Could you check a few things on this drawing? It's one solid part, dimensions in mm from its lowest x, y, z. A direction names the side the tool comes from. Coordinates: 2 decimals unless noted, no trailing zeros. Write each loop counter-clockwise with the first axis right and the second up, starting at its lowest first coordinate (ties: lowest second). Pieces come first, ordered by that corner, then holes. Notation, with made-up numbers: M -1,32.25 L 4,32.25 A27 ccw 4,67.25 Z; hole C -16,-40 d2. An arc over 180 degrees is marked long. Use a Markdown table: item, result.
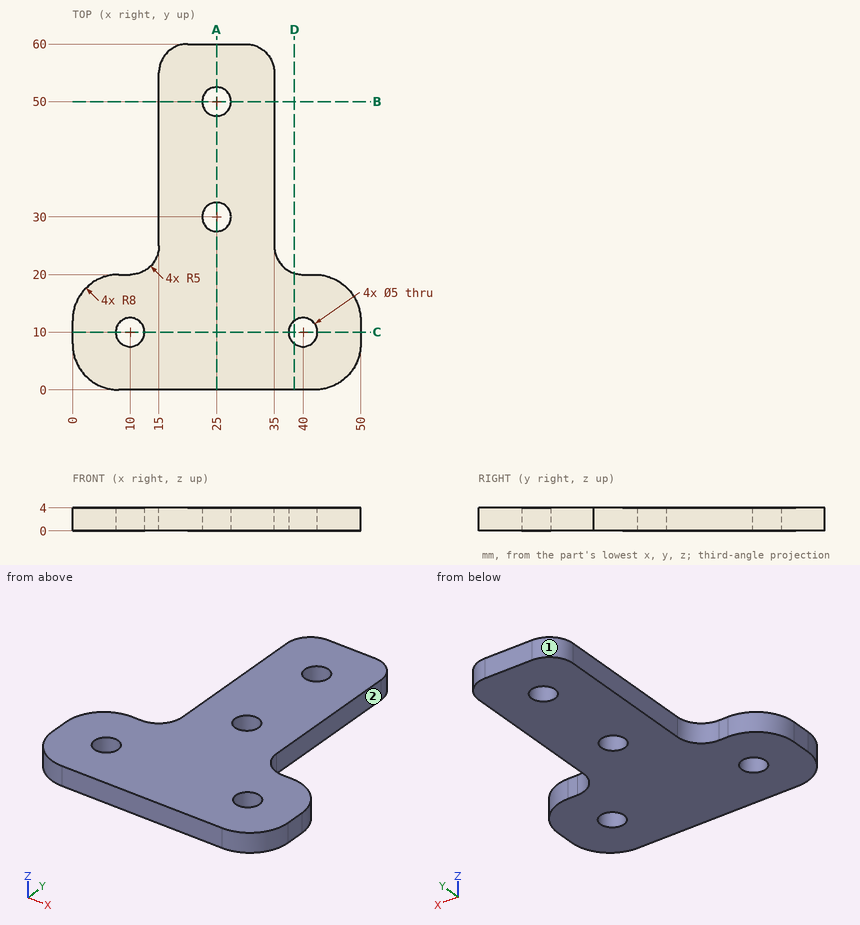
1. Suppose I cut it at B-B on y = 50. Write out the boundary of the cut face in (x, z), and give its area (3 significant figures).
Answers follow:
| item | result |
|---|---|
| outline | M 15,0 L 22.5,0 L 22.5,4 L 15,4 Z; M 27.5,0 L 35,0 L 35,4 L 27.5,4 Z |
| area | 60.0 mm2 |
2. Suppose I cut it at D-D on x = 38.5. Write out the boundary of the cut face in (y, z), and give its area (3 significant figures).
Answers follow:
| item | result |
|---|---|
| outline | M 0,0 L 8,0 L 8,4 L 0,4 Z; M 12,0 L 20.23,0 L 20.23,4 L 12,4 Z |
| area | 64.9 mm2 |
3. Which directions (+Z, -Z, +X, -X, +Y, -Y) give clear straight access to the entire face, cutting with the end or side of a thin tool? Please do the marked faces 1 and 2.
Answers follow:
| item | result |
|---|---|
| face 1 | +Z, -Z, -X, +Y |
| face 2 | +Z, -Z, +X, +Y |
4. Suppose I cut it at A-A on x = 25. Write out the boundary of the cut face in (y, z), and give its area (3 significant figures).
Answers follow:
| item | result |
|---|---|
| outline | M 0,0 L 27.5,0 L 27.5,4 L 0,4 Z; M 32.5,0 L 47.5,0 L 47.5,4 L 32.5,4 Z; M 52.5,0 L 60,0 L 60,4 L 52.5,4 Z |
| area | 200 mm2 |
5. I need wall thicknesses on probe 1 along Y at (x, z) = (25, 1.7); probe 2 along X at (y, z) = (25, 1.2); probe 3 along Y at (x, z) = (38, 1.65). Which ranges of each line are inside material? Lowest first, please.
Answers follow:
| item | result |
|---|---|
| probe 1 | y = 0 to 27.5, 32.5 to 47.5, 52.5 to 60 |
| probe 2 | x = 15 to 35 |
| probe 3 | y = 0 to 8.5, 11.5 to 20.42 |
6. Will these pins go through, and if not, where does the flat tip stop? pin 1 Ø4.5 at (x, y) = (10, 10) entering from -Z; pin 2 Ø0.6 at (x, z) = (8.5, 1) entering from +Y; pin 3 Ø2 at (y, z) = (39.5, 1.5) entering from +X.
Answers follow:
| item | result |
|---|---|
| pin 1 | passes through |
| pin 2 | stops at y = 20 |
| pin 3 | stops at x = 35 |
7. Suppose I cut it at C-C on y = 10. Write out the boundary of the cut face in (x, z), and give its area (3 significant figures).
Answers follow:
| item | result |
|---|---|
| outline | M 0,0 L 7.5,0 L 7.5,4 L 0,4 Z; M 12.5,0 L 37.5,0 L 37.5,4 L 12.5,4 Z; M 42.5,0 L 50,0 L 50,4 L 42.5,4 Z |
| area | 160 mm2 |
